For this review, take the finished solid that the model builds, in its own axes (mm). Face numbers are marked on the shaded views. A direction names the side the tool comes from. Coordinates: 2 decimals unless noted, no trailing zeros. Write each loop counter-clockwise with the first axis right and the second up, starting at its lowest first coordinate (ties: lowest second). Pieces come first, ordered by that corner, then holes.
```python
from build123d import *

# Parameters (mm, degrees)
SKETCH1_W               = 12.7
SKETCH1_H               = 127
BOSS_EXTRUDE1_DEPTH     = 146.05
SKETCH3_R               = 3.175
SKETCH3_R_2             = 12.7
SKETCH3_R_3             = 2.54
CUT_EXTRUDE1_DEPTH      = 12.7
SKETCH4_W               = 25.4
SKETCH4_H               = 127
BOSS_EXTRUDE2_DEPTH     = 6.35
SKETCH9_R               = 3.175
CUT_EXTRUDE2_DEPTH      = 194.961059236
F_1_4_20_TAPPED_HOLE1_D = 5.1054
F_1_4_20_TAPPED_HOLE2_D = 5.1054


with BuildPart() as part:
    # Sketch1 → Boss-Extrude1 (new body)
    with BuildSketch(Plane.XY):
        with Locations((6.35, 63.5)):
            Rectangle(SKETCH1_W, SKETCH1_H)
    extrude(amount=BOSS_EXTRUDE1_DEPTH)

    # Sketch3 → Cut-Extrude1 (cut)
    with BuildSketch(Plane(origin=(12.7, 0, 0), x_dir=(0, 0, -1), z_dir=(1, 0, 0))):
        with Locations((-133.35, 63.5)):
            Circle(SKETCH3_R)
        with Locations((-133.35, 101.6)):
            Circle(SKETCH3_R)
        with Locations((-50.8, 63.5)):
            Circle(SKETCH3_R_2)
        with Locations((-73.914, 86.487)):
            Circle(SKETCH3_R_3)
        with Locations((-27.686, 86.487)):
            Circle(SKETCH3_R_3)
        with Locations((-27.686, 40.513)):
            Circle(SKETCH3_R_3)
        with Locations((-73.914, 40.513)):
            Circle(SKETCH3_R_3)
    extrude(amount=-CUT_EXTRUDE1_DEPTH, mode=Mode.SUBTRACT)

    # Sketch4 → Boss-Extrude2 (add)
    with BuildSketch(Plane.ZY):
        with Locations((133.35, 63.5)):
            Rectangle(SKETCH4_W, SKETCH4_H)
    extrude(amount=BOSS_EXTRUDE2_DEPTH)

    # Sketch9 → Cut-Extrude2 (cut, through all)
    with BuildSketch(Plane(origin=(0, 0, 0), x_dir=(0, 0, -1), z_dir=(1, 0, 0))):
        with Locations((-133.35, 101.6)):
            Circle(SKETCH9_R)
        with Locations((-133.35, 63.5)):
            Circle(SKETCH9_R)
    extrude(amount=-CUT_EXTRUDE2_DEPTH, mode=Mode.SUBTRACT)

    # 1/4-20 Tapped Hole1 (through all)
    with Locations(Plane.ZY):
        with Locations((11.1125, 114.3), (11.1125, 12.7)):
            Hole(F_1_4_20_TAPPED_HOLE1_D / 2)

    # 1/4-20 Tapped Hole2 (through all)
    with Locations(Plane.ZY.offset(6.35)):
        with Locations((134.9375, 114.3), (134.9375, 88.9), (134.9375, 38.1), (134.9375, 12.7)):
            Hole(F_1_4_20_TAPPED_HOLE2_D / 2)


solid = part.part
```
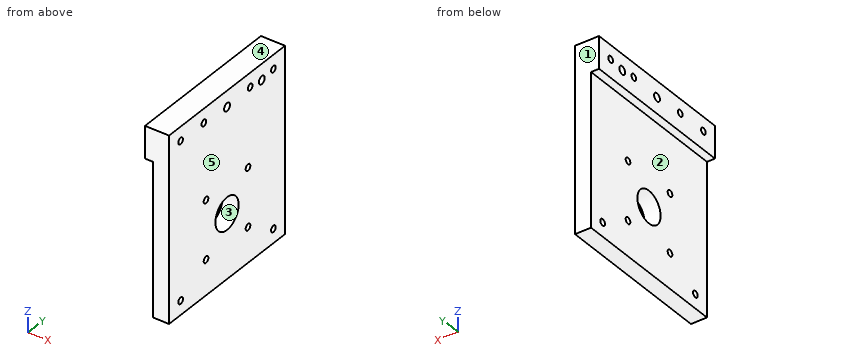
1) Consider section B-B (z = 50.8). Give the boundary of the cut face in (x, y).
2) The part is to be moulded in two halves that separate along Z. For the marked faces 3, 4 and 5, say which applies: pulls with the +Z half, pulls with the -Z half, needs draft (parallel to the pull), parting line crosses it, or undercut.
3) Clearance check with flat-ended pins moving along their axes: P1, Ø5, axis at x = -4, y = 85, coming from the -Z side; P2, Ø6, axis at y = 114.3, z = 134.94, coming from the +X side; P3, Ø5.5, axis at y = 101.6, z = 133.35, coming from the -X side; P4, Ø6.5, axis at y = 40.513, z = 73.914, coming from the -X side. State where each tip first meets the part, or that it passes through.
4) For L1, parallel to Z at x = 1.5, y = 64; L2, parallel to Z at x = 7, y = 14.5; L3, parallel to Z at x = -0.75, y = 43, list the stretches that pass through material, from the lowest coordinate up.
5) Tool access review of the marked faces 1 and 2: name each direction out of +Z, -Z, +X, -X, +Y, -Y from which nothing blocks a thin tool from reaching the whole face with its end or side.
6) Consider section D-D (y = 63.5). Give the boundary of the cut face in (x, z) (3 decimals).
7) Consider section C-C (x = -3.5). Count the separate pieces of the cut face and the enclosed holes in it, then the cut area to 3 significant figures.
8) Consider section A-A (y = 12.7). Give the boundary of the cut face in (x, z).
Results:
1. outline: (0, 0) - (12.7, 0) - (12.7, 50.8) - (0, 50.8) - close; (0, 76.2) - (12.7, 76.2) - (12.7, 127) - (0, 127) - close
2. face 3: undercut
2. face 4: pulls with the +Z half
2. face 5: needs draft
3. P1: stops at z = 120.65
3. P2: stops at x = 12.7
3. P3: passes through
3. P4: stops at x = 0
4. L1: z = 0 to 38.11, 63.49 to 130.21, 136.49 to 146.05
4. L2: z = 0 to 9.3, 12.92 to 133.13, 136.75 to 146.05
4. L3: z = 120.65 to 146.05
5. face 1: +Z, -Z, +X, -X, +Y
5. face 2: -Z, -X, +Y, -Y
6. outline: (-6.35, 120.65) - (0, 120.65) - (0, 63.5) - (12.7, 63.5) - (12.7, 130.175) - (-6.35, 130.175) - close; (-6.35, 136.525) - (12.7, 136.525) - (12.7, 146.05) - (-6.35, 146.05) - close; (0, 0) - (12.7, 0) - (12.7, 38.1) - (0, 38.1) - close
7. separate pieces: 1
7. enclosed holes: 6
7. area: 3,080 mm2
8. outline: (-6.35, 120.65) - (0, 120.65) - (0, 13.67) - (12.7, 13.67) - (12.7, 132.38) - (-6.35, 132.38) - close; (-6.35, 137.49) - (12.7, 137.49) - (12.7, 146.05) - (-6.35, 146.05) - close; (0, 0) - (12.7, 0) - (12.7, 8.56) - (0, 8.56) - close
